Could you check a few things on this model? Use its own coordinates, in mm. A direction names the side the tool comes from. Give positions to 0.01 mm unless a question says otherwise; leave off trailing zeros. Write each loop counter-clockwise with the first axis right and the second up, starting at its lowest first coordinate (ties: lowest second). Pieces come first, ordered by that corner, then holes. Notation, with made-up numbers: (-13, -17) - (19, -17) arc R23 cw to (19, -1) - close; hole circle Ø5 at (60.5, 15.25). An arc over 180 degrees is marked (long way). Answer in a Markdown table with one row per item.
from build123d import *

# Parameters (mm, degrees)
CHAMFER_1_SIZE = 0.5


with BuildPart() as part:
    # 草图1 → 旋转1 (revolve)
    with BuildSketch(Plane(origin=(0, 0, 0), x_dir=(1, 0, 0), z_dir=(0, 1, 0)), mode=Mode.PRIVATE) as revolve_1_sk:
        with BuildLine():
            Line((-12.5, 7), (12.5, 7))
            Line((12.5, 7), (12.5, 6.4))
            Line((12.5, 6.4), (13, 6.4))
            ThreePointArc((13, 6.4), (13.594102968, 6.225765447), (14, 5.758257569))
            Line((14, 5.758257569), (14, 5.5))
            Line((14, 5.5), (15.5, 5.5))
            Line((15.5, 5.5), (15.5, 4.5))
            Line((15.5, 4.5), (16.5, 4.5))
            Line((16.5, 4.5), (16.5, 6.25))
            Line((16.5, 6.25), (18.5, 6.25))
            Line((18.5, 6.25), (18.5, 3))
            Line((18.5, 3), (-18.5, 3))
            Line((-18.5, 3), (-18.5, 6.25))
            Line((-18.5, 6.25), (-16.5, 6.25))
            Line((-16.5, 6.25), (-16.5, 4.5))
            Line((-16.5, 4.5), (-15.5, 4.5))
            Line((-15.5, 4.5), (-15.5, 5.5))
            Line((-15.5, 5.5), (-14, 5.5))
            Line((-14, 5.5), (-14, 5.758257569))
            ThreePointArc((-14, 5.758257569), (-13.594102968, 6.225765447), (-13, 6.4))
            Line((-13, 6.4), (-12.5, 6.4))
            Line((-12.5, 6.4), (-12.5, 7))
        make_face()
    revolve(revolve_1_sk.sketch.rotate(Axis((-37.377186512, 0, 0), (1, 0, 0)), 180), axis=Axis((-37.377186512, 0, 0), (1, 0, 0)))

    # 倒角1
    chamfer_1_edges = [part.edges().sort_by_distance(p)[0] for p in [
        (-12.5, 0, -7),
        (12.5, 0, -7),
    ]]
    chamfer(chamfer_1_edges, length=CHAMFER_1_SIZE)


solid = part.part
1) Imagine slicing it at A-A (x = -4.5). List the corners of the cut face in (y, z) for me, then the cut area to 3 significant figures.
Check values:
| item | result |
|---|---|
| outline | circle Ø14 at (0, 0); hole circle Ø6 at (0, 0) |
| area | 126 mm2 |
2) Will these pins go through, and if not, where does the flat tip stop? P1, Ø5, axis at x = -2, z = -4, coming from the +Y side; P2, Ø4, axis at x = -12.5, y = 5.5, coming from the -Z side; P3, Ø5, axis at x = 9, z = 5, coming from the -Y side.
Check values:
| item | result |
|---|---|
| P1 | stops at y = 6.84 |
| P2 | stops at z = -6.03 |
| P3 | stops at y = -6.54 |
3) If I drill on line 1 (X direction, y = 4.75, z = -0.75); line 2 (X direction, y = -2, z = -5.75); line 3 (Y direction, x = 5, z = 0), over which ranges is the centre line in solid material (lowest first)?
Check values:
| item | result |
|---|---|
| line 1 | x = -18.5 to -16.5, -15.5 to 15.5, 16.5 to 18.5 |
| line 2 | x = -18.5 to -16.5, -13.77 to 13.77, 16.5 to 18.5 |
| line 3 | y = -7 to -3, 3 to 7 |
4) We'd pull the mould along X, two halves only. Please class faces 5 (the face through (-18.5, 3, 1)), 6 (the face through (16.5, 4, -3)), 7 (the face through (-17.49, -1.88, 5.96)): +X half, -X half, draft (parallel to the pull), parting line (faces both ways), or undercut.
Check values:
| item | result |
|---|---|
| face 5 | -X half |
| face 6 | undercut |
| face 7 | draft |
5) Imagine slicing it at B-B (x = -15). List the corners of the cut face in (y, z) for me.
Check values:
| item | result |
|---|---|
| outline | circle Ø11 at (0, 0); hole circle Ø6 at (0, 0) |
6) On a 3-axis mill with a long thin cutter (end or side, diameter ignored), from which of +Z, -Z, +X, -X, +Y, -Y can I reach the whole of each face in a straight line? I mean faces 1 (the face through (15.5, 0, -5)), 2 (the face through (-12.746, -1.922, 6.104)), 3 (the face through (17.51, -1.88, 5.96)), 4 (the face through (0.168, 2.681, 6.466)). Say none if no direction works.
Check values:
| item | result |
|---|---|
| face 1 | none |
| face 2 | -X |
| face 3 | +X |
| face 4 | +X, -X |
